Can you work these out from the model? Positions are in its coordinate system, mm. A direction names the side the tool comes from. Round coordinates to 2 decimals unless told otherwise and drop trailing zeros. Write each loop counter-clockwise with the first axis right and the second up, starting at its lowest first coordinate (ties: lowest second). Pieces come first, ordered by that corner, then holes.
Q1. For faces 3 (the flat face through (-24, 0, -502)), 4 (the flat face through (-19, -3, -542)), which set-ups out of +Z, -Z, +X, -X, +Y, -Y let a thin tool reach every point of the face, with its end or its side?
Q2. If we section it at A-A (z = -698.5): Please give me the cut outline in (x, y), plus the area to 3 significant figures.
Q3. If we section it at B-B (x = 199): Please give me the cut outline in (y, z), plus the area to 3 significant figures.
Q4. We'd pull the mould along X, two halves only. Please class faces 1 (the flat face through (-19, -13, -542)), 2 (the flat face through (-24, -16, -502)): +X half, -X half, draft (parallel to the pull), parting line (faces both ways), or undercut.
Q5. I'm going to push flat-ended pins straight in: pin 1 Ø16 at (x, z) = (300, -1017) entering from -Y; pin 2 Ø6 at (x, z) = (300, 17) entering from +Y. Where does each tip first touch, or does it pass through?
Q6. Please list where these lines run through material, in increasing order: line 1 along Z through (x, y) = (300, -14.45); line 2 along X through (y, z) = (-15.25, -406); line 3 along Z through (x, y) = (514.5, -13.75).
from build123d import *

# Parameters (mm, degrees)
SWEEP_START           = -16
SWEEP_1_OUTLINE_W     = 670
SWEEP_1_OUTLINE_H     = 1070
SWEEP_1_OUTLINE_W_2   = 600
SWEEP_1_OUTLINE_H_2   = 1000
SWEEP_1_DEPTH         = 3
SWEEP_START_2         = -3
SWEEP_1_2_OUTLINE_W   = 670
SWEEP_1_2_OUTLINE_H   = 1070
SWEEP_1_2_OUTLINE_W_2 = 600
SWEEP_1_2_OUTLINE_H_2 = 1000
SWEEP_1_2_DEPTH       = 3
SWEEP_START_3         = -13
SWEEP_1_3_OUTLINE_W   = 670
SWEEP_1_3_OUTLINE_H   = 1070
SWEEP_1_3_OUTLINE_W_2 = 660
SWEEP_1_3_OUTLINE_H_2 = 1060
SWEEP_1_3_DEPTH       = 10
SKETCH_16_R           = 3
CUT_EXTRUDE_1_DEPTH   = 1245.339583876
SKETCH_17_R           = 5
CUT_EXTRUDE_2_DEPTH   = 1215.374736233


# Read off the part's stored shape, not the designer's step: 扫描1
with BuildPart() as part:
    # 扫描1 outline → 扫描1 (new body)
    with BuildSketch(Plane(origin=(0, 0, 0), x_dir=(1, 0, 0), z_dir=(0, 1, 0)).offset(SWEEP_START)):
        with Locations((300, 500)):
            Rectangle(SWEEP_1_OUTLINE_W, SWEEP_1_OUTLINE_H)
        with Locations((300, 500)):
            Rectangle(SWEEP_1_OUTLINE_W_2, SWEEP_1_OUTLINE_H_2, mode=Mode.SUBTRACT)
    extrude(amount=SWEEP_1_DEPTH)



with BuildPart() as body_2:
    # Sweep 1 2 outline → Sweep 1 2 (new body)
    with BuildSketch(Plane(origin=(0, 0, 0), x_dir=(1, 0, 0), z_dir=(0, 1, 0)).offset(SWEEP_START_2)):
        with Locations((300, 500)):
            Rectangle(SWEEP_1_2_OUTLINE_W, SWEEP_1_2_OUTLINE_H)
        with Locations((300, 500)):
            Rectangle(SWEEP_1_2_OUTLINE_W_2, SWEEP_1_2_OUTLINE_H_2, mode=Mode.SUBTRACT)
    extrude(amount=SWEEP_1_2_DEPTH)


with BuildPart() as part_1:
    add(part.part)

    add(body_2.part)  # Sweep 1 3 merges body 2
    # Sweep 1 3 outline → Sweep 1 3 (add)
    with BuildSketch(Plane(origin=(0, 0, 0), x_dir=(1, 0, 0), z_dir=(0, 1, 0)).offset(SWEEP_START_3)):
        with Locations((300, 500)):
            Rectangle(SWEEP_1_3_OUTLINE_W, SWEEP_1_3_OUTLINE_H)
        with Locations((300, 500)):
            Rectangle(SWEEP_1_3_OUTLINE_W_2, SWEEP_1_3_OUTLINE_H_2, mode=Mode.SUBTRACT)
    extrude(amount=SWEEP_1_3_DEPTH)

    # 草图16 → 切除-拉伸1 (cut, through all)
    with BuildSketch(Plane.XY.offset(35)):
        with Locations((-17, -8)):
            Circle(SKETCH_16_R)
    extrude(amount=-CUT_EXTRUDE_1_DEPTH, mode=Mode.SUBTRACT)

    # 草图17 → 切除-拉伸2 (cut, through all)
    with BuildSketch(Plane(origin=(0, 0, 0), x_dir=(1, 0, 0), z_dir=(0, 1, 0))):
        with Locations(Location((300, 1017, 0), (0, 0, 270))):
            Circle(SKETCH_17_R)
        with Locations(Location((300, -17, 0), (0, 0, 270))):
            Circle(SKETCH_17_R)
    extrude(amount=-CUT_EXTRUDE_2_DEPTH, mode=Mode.SUBTRACT)


solid = part_1.part
A:
1. face 3: +Z, -Z, +X, -X, +Y
1. face 4: none
2. outline: (-35, -16) - (0, -16) - (0, -13) - (-30, -13) - (-30, -3) - (0, -3) - (0, 0) - (-35, 0) - close; (600, -16) - (635, -16) - (635, 0) - (600, 0) - (600, -3) - (630, -3) - (630, -13) - (600, -13) - close
2. area: 520 mm2
3. outline: (-16, -1035) - (0, -1035) - (0, -1000) - (-3, -1000) - (-3, -1030) - (-13, -1030) - (-13, -1000) - (-16, -1000) - close; (-16, 0) - (-13, 0) - (-13, 30) - (-3, 30) - (-3, 0) - (0, 0) - (0, 35) - (-16, 35) - close
3. area: 520 mm2
4. face 1: undercut
4. face 2: draft
5. pin 1: stops at y = -16
5. pin 2: passes through
6. line 1: z = -1035 to -1022, -1012 to -1000, 0 to 12, 22 to 35
6. line 2: x = -35 to 0, 600 to 635
6. line 3: z = -1035 to -1000, 0 to 35
